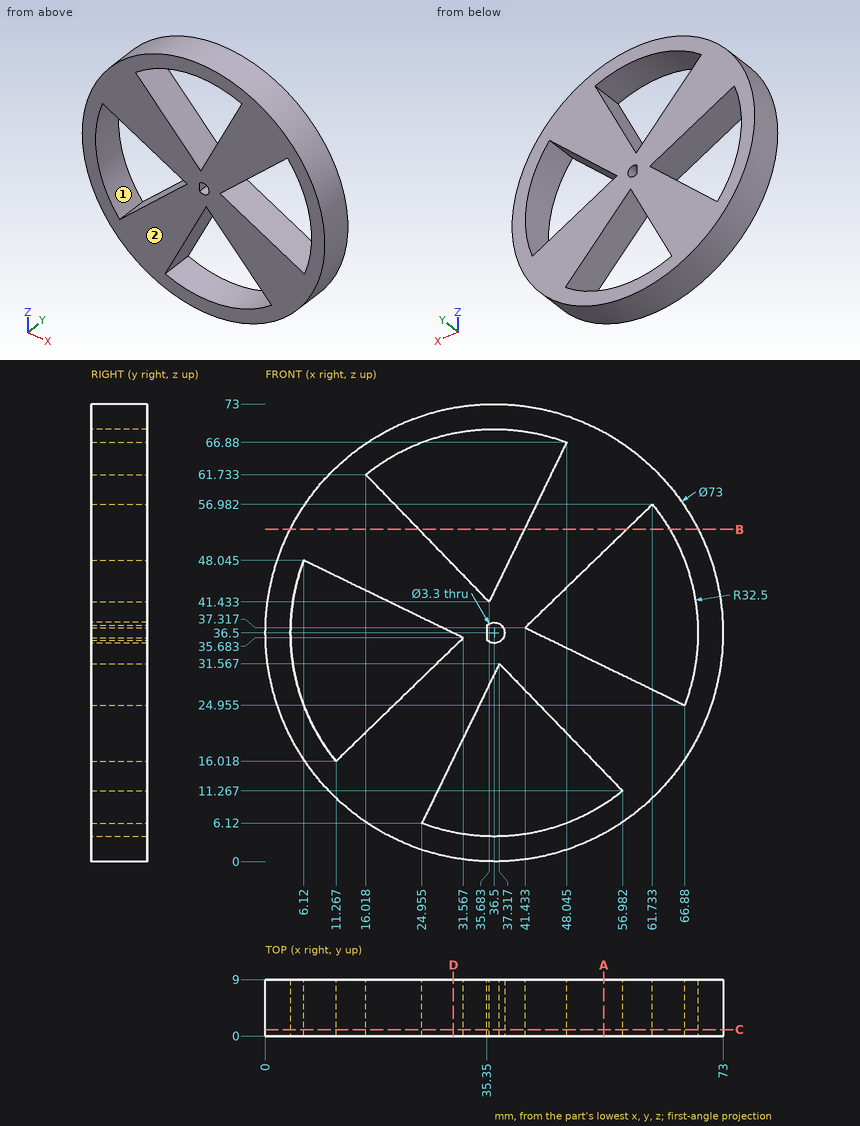
Geometry: see drawing. Coordinates: mm, zero at the bounding-box minimum. A direction names the side the tool comes from. Give positions to 0.01 mm unless a question says otherwise; leave off trailing zeros. Order: outer loops, then holes, each group sorted by start corner. A loop starts at its lowest first (then second) coordinate and runs counter-clockwise, first axis right, second up. Notation, with made-up numbers: M 45,52 L 67,52 A24 cw 67,77 Z; hole C -19.5,-9 d3. An arc over 180 degrees is marked long. Answer as CSV lines item,"result". Start each with the question number.
1) Cut plane D-D (x = 30). Output: boundary loops of the cut face in (y, z) (1 decimal).
2) Set-up query: the marked faces 1 and 2. Return all of +Z, -Z, +X, -X, +Y, -Y with unobstructed straight access to the full face (end or side cutting, diameter ignored); none if empty.
3) Cut plane A-A (x = 54). Output: boundary loops of the cut face in (y, z) (1 decimal), then the cut area to 3 significant figures.
4) First-contact query: P1, Ø6, axis at x = 65, z = 37, coming from the +Y side; P2, Ø5, axis at x = 43.5, y = 6.5, coming from the -Z side; P3, Ø4, axis at x = 17.5, y = 4.5, coming from the +Z side; P4, Ø5, axis at x = 18.5, y = 1.5, coming from the +Z side (1 decimal). Flat tips, straight axial feed; report the tip coordinate or a pass-through.
5) Cut plane C-C (y = 1). State how many separate pieces and enclosed holes the cut face has, then the cut area to 3 significant figures.
6) Line query: line 1 (X direction, y = 1, z = 45) (1 decimal); line 2 (X direction, y = 1.25, z = 22.5); line 3 (X direction, y = 6.5, z = 20.5) (1 decimal). Output: solid intervals per line, ascending. Write a range as from..to.
7) Cut plane B-B (z = 53). Output: boundary loops of the cut face in (x, y).
Findings below:
1,outline,"M 0,0.6 L 9,0.6 L 9,4.7 L 0,4.7 Z; M 0,16.5 L 9,16.5 L 9,34.2 L 0,34.2 Z; M 0,36.4 L 9,36.4 L 9,47.3 L 0,47.3 Z; M 0,68.3 L 9,68.3 L 9,72.4 L 0,72.4 Z"
2,face 1,"+Y, -Y"
2,face 2,"+Z, -Z, +X, -X, -Y"
3,outline,"M 0,4.5 L 9,4.5 L 9,9.1 L 0,9.1 Z; M 0,14.3 L 9,14.3 L 9,31.2 L 0,31.2 Z; M 0,49.5 L 9,49.5 L 9,68.5 L 0,68.5 Z"
3,area,"365 mm²"
4,P1,"passes through"
4,P2,"stops at z = 0.28"
4,P3,"stops at z = 68.8"
4,P4,"stops at z = 69.5"
5,separate pieces,"1"
5,enclosed holes,"5"
5,area,"2,290 mm²"
6,line 1,"x = 1..5.1, 12.4..32.2, 37.4..49.4, 67.9..72"
6,line 2,"x = 2.79..7.17, 17.96..32.91, 46.1..70.21"
6,line 3,"x = 3.7..8.2, 15.9..31.9, 48..69.3"
7,outline,"M 3.94,0 L 24.48,0 L 24.48,9 L 3.94,9 Z; M 41.3,0 L 57.62,0 L 57.62,9 L 41.3,9 Z; M 64.5,0 L 69.06,0 L 69.06,9 L 64.5,9 Z"
